Geometry check sheet. Reference: the model listing, model coordinates, mm. Face numbers are marked on the shaded views. A direction names the side the tool comes from. Round coordinates to 2 decimals unless told otherwise and drop trailing zeros. Loops run counter-clockwise (first coordinate to the right, second up) from the corner with the lowest first, then second, coordinate; pieces in that order, holes last. Notation, with made-up numbers: M 19.5,-10 L 46.5,-10 A20 cw 46.5,28 Z; hole C -34,42.5 d4. An arc over 180 degrees is marked long. Write item = value, one per line.
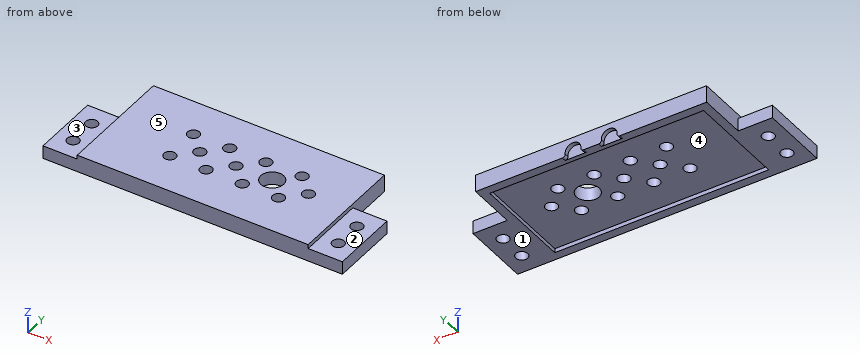
from build123d import *

# Parameters (mm, degrees)
SKETCH1_W           = 81
SKETCH1_H           = 41
BOSS_EXTRUDE1_DEPTH = 6
SKETCH5_W           = 75
SKETCH5_H           = 35
CUT_EXTRUDE1_DEPTH  = 1.43
SKETCH8_R           = 2.1
SKETCH8_R_2         = 4
CUT_EXTRUDE2_DEPTH  = 7
SKETCH9_R           = 2.75
CUT_EXTRUDE3_DEPTH  = 1.5
FILLET1_R           = 1
SKETCH10_W          = 4.57
SKETCH10_H          = 24
BOSS_EXTRUDE2_DEPTH = 12
SKETCH12_W          = 4.57
SKETCH12_H          = 24
BOSS_EXTRUDE3_DEPTH = 12
SKETCH13_R          = 2.1
CUT_EXTRUDE4_DEPTH  = 5.57


with BuildPart() as part:
    # Sketch1 → Boss-Extrude1 (new body)
    with BuildSketch(Plane.XY):
        Rectangle(SKETCH1_W, SKETCH1_H)
    extrude(amount=BOSS_EXTRUDE1_DEPTH)

    # Sketch5 → Cut-Extrude1 (cut)
    with BuildSketch(Plane(origin=(0, 0, 0), x_dir=(-1, 0, 0), z_dir=(0, 0, -1))):
        Rectangle(SKETCH5_W, SKETCH5_H)
    extrude(amount=-CUT_EXTRUDE1_DEPTH, mode=Mode.SUBTRACT)

    # Sketch8 → Cut-Extrude2 (cut, through all)
    with BuildSketch(Plane.XY.offset(6)):
        with Locations((26.9, 0.5)):
            Circle(SKETCH8_R)
        with Locations((20.55, 6.849637785)):
            Circle(SKETCH8_R)
        with Locations((7.85, 6.849637785)):
            Circle(SKETCH8_R)
        with Locations((7.85, -5.849637785)):
            Circle(SKETCH8_R)
        with Locations((20.55, -5.849637785)):
            Circle(SKETCH8_R)
        with Locations((1.5, 0.5)):
            Circle(SKETCH8_R)
        with Locations((-4.85, 6.849637785)):
            Circle(SKETCH8_R)
        with Locations((-4.85, -5.849637785)):
            Circle(SKETCH8_R)
        with Locations((-11.2, 0.5)):
            Circle(SKETCH8_R)
        with Locations((-17.55, 6.849637785)):
            Circle(SKETCH8_R)
        with Locations((-17.55, -5.849637785)):
            Circle(SKETCH8_R)
        with Locations((14.2, 0.5)):
            Circle(SKETCH8_R_2)
    extrude(amount=-CUT_EXTRUDE2_DEPTH, mode=Mode.SUBTRACT)

    # Sketch9 → Cut-Extrude3 (cut)
    with BuildSketch(Plane(origin=(0, 20.5, 0), x_dir=(1, 0, 0), z_dir=(0, 1, 0))):
        with Locations((6.35, -1.35)):
            Circle(SKETCH9_R)
        with Locations((-6.35, -1.35)):
            Circle(SKETCH9_R)
    extrude(amount=-CUT_EXTRUDE3_DEPTH, mode=Mode.SUBTRACT)

    # Fillet1
    fillet1_edges = [part.edges().sort_by_distance(p)[0] for p in [
        (-8.74582971, 19.75, 0),
        (-3.95417029, 19.75, 0),
        (3.95417029, 19.75, 0),
        (8.74582971, 19.75, 0),
    ]]
    fillet(fillet1_edges, radius=FILLET1_R)

    # Sketch10 → Boss-Extrude2 (add)
    with BuildSketch(Plane.ZY.offset(40.5)):
        with Locations((2.285, -8.5)):
            Rectangle(SKETCH10_W, SKETCH10_H)
    extrude(amount=BOSS_EXTRUDE2_DEPTH)

    # Sketch12 → Boss-Extrude3 (add)
    with BuildSketch(Plane(origin=(40.5, 0, 0), x_dir=(0, 0, -1), z_dir=(1, 0, 0))):
        with Locations((-2.285, -8.5)):
            Rectangle(SKETCH12_W, SKETCH12_H)
    extrude(amount=BOSS_EXTRUDE3_DEPTH)

    # Sketch13 → Cut-Extrude4 (cut, through all)
    with BuildSketch(Plane.XY.offset(4.57)):
        with Locations((-46.5, -3.5)):
            Circle(SKETCH13_R)
        with Locations((-46.5, -13.5)):
            Circle(SKETCH13_R)
        with Locations((46.5, -3.5)):
            Circle(SKETCH13_R)
        with Locations((46.5, -13.5)):
            Circle(SKETCH13_R)
    extrude(amount=-CUT_EXTRUDE4_DEPTH, mode=Mode.SUBTRACT)


solid = part.part
(1) Sectioned sample at C-C on y = 0.5. Record the cut outline in (x, z).
Result set:
outline = M -52.5,0 L -37.5,0 L -37.5,1.43 L -13.3,1.43 L -13.3,6 L -40.5,6 L -40.5,4.57 L -52.5,4.57 Z; M -9.1,1.43 L -0.6,1.43 L -0.6,6 L -9.1,6 Z; M 3.6,1.43 L 10.2,1.43 L 10.2,6 L 3.6,6 Z; M 18.2,1.43 L 24.8,1.43 L 24.8,6 L 18.2,6 Z; M 29,1.43 L 37.5,1.43 L 37.5,0 L 52.5,0 L 52.5,4.57 L 40.5,4.57 L 40.5,6 L 29,6 Z
(2) Release check for a two-part mould opening along X. For the marked faces 4 and 5 record: released by +X, released by -X, zero draft, split by the parting line, or undercut.
Result set:
face_4 = undercut
face_5 = zero draft
(3) Sectioned sample at A-A on x = 20.55. Record the cut outline in (y, z).
Result set:
outline = M -20.5,0 L -17.5,0 L -17.5,1.43 L -7.95,1.43 L -7.95,6 L -20.5,6 Z; M -3.75,1.43 L 4.75,1.43 L 4.75,6 L -3.75,6 Z; M 8.95,1.43 L 17.5,1.43 L 17.5,0 L 20.5,0 L 20.5,6 L 8.95,6 Z
(4) Depth check by flat-ended pin: pin 1 Ø5.5 at (x, y) = (-4.85, 6.85) entering from -Z; pin 2 Ø6 at (x, y) = (-46.5, -14) entering from +Z. Enter the tip coordinate at first touch or a pass-through.
Result set:
pin_1 = 1.43
pin_2 = 4.57
(5) Sectioned sample at B-B on y = -13.5. Record the cut outline in (x, z), then the cut area to 3 significant figures.
Result set:
outline = M -52.5,0 L -48.6,0 L -48.6,4.57 L -52.5,4.57 Z; M -44.4,0 L -37.5,0 L -37.5,1.43 L 37.5,1.43 L 37.5,0 L 44.4,0 L 44.4,4.57 L 40.5,4.57 L 40.5,6 L -40.5,6 L -40.5,4.57 L -44.4,4.57 Z; M 48.6,0 L 52.5,0 L 52.5,4.57 L 48.6,4.57 Z
area = 450 mm2
(6) Tool access check on the marked faces 1, 2 and 3. Record the directions out of +Z, -Z, +X, -X, +Y, -Y that give a thin tool (end or side, any length) a straight path to the whole face; none if there is none.
Result set:
face_1 = -Z, +X, -X, +Y, -Y
face_2 = +Z, +X, +Y, -Y
face_3 = +Z, -X, +Y, -Y
(7) Sectioned sample at D-D on x = 1.5. Record the cut outline in (y, z).
Result set:
outline = M -20.5,0 L -17.5,0 L -17.5,1.43 L -1.6,1.43 L -1.6,6 L -20.5,6 Z; M 2.6,1.43 L 17.5,1.43 L 17.5,0 L 20.5,0 L 20.5,6 L 2.6,6 Z
(8) Material ranges on line 1 along Y through (x, z) = (-46.5, 1.5); line 2 along X through (y, z) = (19.9, 1.35); line 3 along Y through (x, z) = (7.85, 4.7), recorded low to high. Write a range as from..to.
Result set:
line_1 = -20.5..-15.6, -11.4..-5.6, -1.4..3.5
line_2 = -40.5..-9.1, -3.6..3.6, 9.1..40.5
line_3 = -20.5..-7.95, -3.75..4.75, 8.95..20.5
